from build123d import *

# Parameters (mm, degrees)
SKETCH1_R           = 2.5
BOSS_EXTRUDE1_DEPTH = 4


with BuildPart() as part:
    # Sketch1 → Boss-Extrude1 (new body)
    with BuildSketch(Plane(origin=(0, 0, 0), x_dir=(1, 0, 0), z_dir=(0, 1, 0))):
        with BuildLine():
            Line((-28.278974074, 16.963626091), (11.721025926, 26.963626091))
            ThreePointArc((11.721025926, 26.963626091), (18.155634684, 25.599098125), (21.040043114, 19.687557339))
            Line((21.040043114, 19.687557339), (21.040043114, -19.687557339))
            ThreePointArc((21.040043114, -19.687557339), (16.927889481, -26.378782712), (9.100710583, -25.732582292))
            Line((9.100710583, -25.732582292), (-30.899289417, 3.642532387))
            ThreePointArc((-30.899289417, 3.642532387), (-33.81893913, 11.1351002), (-28.278974074, 16.963626091))
        make_face()
        with Locations(Location((-26.459956886, 9.687557339, 0), (0, 0, 270))):
            Circle(SKETCH1_R, mode=Mode.SUBTRACT)
        with Locations(Location((-6.459956886, 9.687557339, 0), (0, 0, 270))):
            Circle(SKETCH1_R, mode=Mode.SUBTRACT)
        with Locations(Location((13.540043114, 19.687557339, 0), (0, 0, 270))):
            Circle(SKETCH1_R, mode=Mode.SUBTRACT)
        with Locations(Location((13.540043114, -0.312442661, 0), (0, 0, 90))):
            Circle(SKETCH1_R, mode=Mode.SUBTRACT)
        with Locations(Location((13.540043114, -19.687557339, 0), (0, 0, 270))):
            Circle(SKETCH1_R, mode=Mode.SUBTRACT)
    extrude(amount=BOSS_EXTRUDE1_DEPTH)


solid = part.part
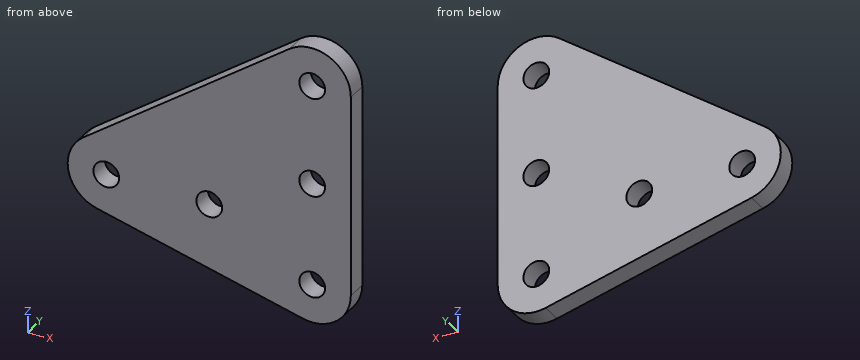
Input: part model. Units: mm. Frame: model coordinates. Coordinates: 2 decimals unless noted, no trailing zeros. Order: outer loops, then holes, each group sorted by start corner. A loop starts at its lowest first (then second) coordinate and runs counter-clockwise, first axis right, second up. Notation, with made-up numbers: M 66.25,62.5 L 96.25,62.5 A29 ccw 96.25,93.5 Z; hole C 68,-9 d9. An arc over 180 degrees is marked long. Answer in a Markdown table with one row per item.
(1) Section query B-B, the plane y = 2.4. Output: boundary loops of the cut face in (x, z), plus the area to 3 significant figures.
Numbers:
| item | result |
|---|---|
| outline | M -30.9,-3.64 A7.5 ccw -28.28,-16.96 L 11.72,-26.96 A7.5 ccw 21.04,-19.69 L 21.04,19.69 A7.5 ccw 9.1,25.73 Z; hole C -26.46,-9.69 d5; hole C -6.46,-9.69 d5; hole C 13.54,-19.69 d5; hole C 13.54,0.31 d5; hole C 13.54,19.69 d5 |
| area | 1,840 mm^2 |
(2) Section query C-C, the plane x = -27.5. Output: boundary loops of the cut face in (y, z), plus the area to 3 significant figures.
Numbers:
| item | result |
|---|---|
| outline | M 0,-17.16 L 4,-17.16 L 4,-11.96 L 0,-11.96 Z; M 0,-7.41 L 4,-7.41 L 4,-1.15 L 0,-1.15 Z |
| area | 45.9 mm^2 |
(3) Section query D-D, the plane z = -8. Output: boundary loops of the cut face in (x, y).
Numbers:
| item | result |
|---|---|
| outline | M -33.77,0 L -28.3,0 L -28.3,4 L -33.77,4 Z; M -24.62,0 L -8.3,0 L -8.3,4 L -24.62,4 Z; M -4.62,0 L 21.04,0 L 21.04,4 L -4.62,4 Z |
(4) Section query A-A, the plane z = 18.5. Output: boundary loops of the cut face in (x, y), plus the area to 3 significant figures.
Numbers:
| item | result |
|---|---|
| outline | M -0.75,0 L 11.34,0 L 11.34,4 L -0.75,4 Z; M 15.74,0 L 21.04,0 L 21.04,4 L 15.74,4 Z |
| area | 69.6 mm^2 |
(5) Material intervals for line 1 (Z direction, x = 15, y = 2.9); line 2 (Z direction, x = 11.5, y = 3.2); line 3 (Z direction, x = -27, y = 1.45), sorted ascending. Write a range as [from, to].
Numbers:
| item | result |
|---|---|
| line 1 | z = [-27.04, -21.72], [-17.66, -1.72], [2.34, 17.66], [21.72, 27.04] |
| line 2 | z = [-26.91, -21.13], [-18.24, -1.13], [1.76, 18.24], [21.13, 26.9] |
| line 3 | z = [-17.28, -12.13], [-7.25, -0.78] |
(6) Contact query for flat-ended pins moving along their axis: pin 1 Ø4.5 at (x, z) = (13.54, 19.69) entering from -Y; pin 2 Ø2 at (y, z) = (2, -16.5) entering from -X; pin 3 Ø8 at (x, z) = (13.54, 0.31) entering from +Y; pin 4 Ø2 at (y, z) = (1.5, -13.5) entering from -X. Output: stop coordinate, or through.
Numbers:
| item | result |
|---|---|
| pin 1 | passes through |
| pin 2 | stops at x = -31.2 |
| pin 3 | stops at y = 4 |
| pin 4 | stops at x = -33.41 |
